Part model, mm, in its own coordinate system. Coordinates: 2 decimals unless noted, no trailing zeros. Write each loop counter-clockwise with the first axis right and the second up, starting at its lowest first coordinate (ties: lowest second). Pieces come first, ordered by that corner, then holes. Notation, with made-up numbers: (27, 30.5) - (56, 30.5) arc R15 cw to (56, 50.5) - close; hole circle Ø10 at (83.5, 61.5). An arc over 180 degrees is marked (long way). Use a Markdown table: item, result.
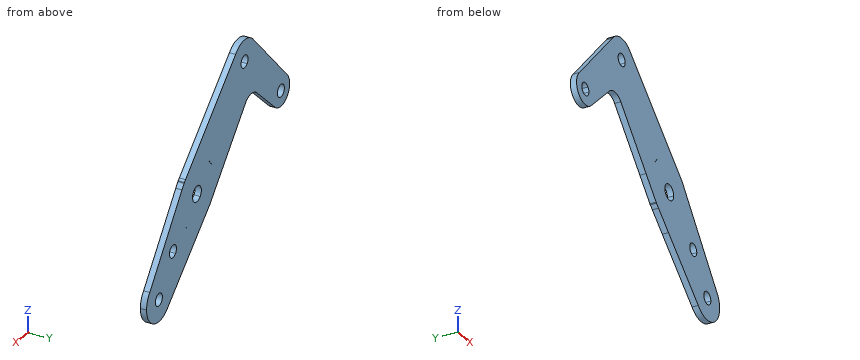
```python
from build123d import *

# Parameters (mm, degrees)
F1_DEPTH = 3.175


with BuildPart() as f1:
    # F0 (on Front) → F1 (new body)
    with BuildSketch(Plane.XZ):
        with BuildLine():
            ThreePointArc((-2.6877932952, 2.9286835289), (1.5995582019, 3.6390704265), (3.9751, 0))
            ThreePointArc((3.9751, 0), (3.6390704265, -1.5995582019), (2.6877932952, -2.9286835289))
            Line((2.6877932952, -2.9286835289), (10.7339987827, -11.6960204828))
            ThreePointArc((10.7339987827, -11.6960204828), (14.5330288597, -6.3880119883), (15.875, 0))
            ThreePointArc((15.875, 0), (15.2734304328, 4.3287351287), (13.5143136611, 8.3294028158))
            Line((13.5143136611, 8.3294028158), (11.6590601378, 10.7741329908))
            Line((11.6590601378, 10.7741329908), (11.4851871667, 10.9592928944))
            Line((11.4851871667, 10.9592928944), (11.3083739877, 11.1416472191))
            Line((11.3083739877, 11.1416472191), (10.3225973322, 12.0606637179))
            ThreePointArc((10.3225973322, 12.0606637179), (-0.2748708071, 15.8726201693), (-10.7339987827, 11.6960204828))
            Line((-10.7339987827, 11.6960204828), (-2.6877932952, 2.9286835289))
        make_face()
        with BuildLine():
            ThreePointArc((-2.9286835289, -2.6877932952), (-3.9714488487, 0.1703351178), (-2.6877932952, 2.9286835289))
            Line((-2.6877932952, 2.9286835289), (-10.7339987827, 11.6960204828))
            Line((-10.7339987827, 11.6960204828), (-13.3268527784, 8.6261590538))
            ThreePointArc((-13.3268527784, 8.6261590538), (-15.8291292061, -1.2059409505), (-11.8662618768, -10.5454944915))
            Line((-11.8662618768, -10.5454944915), (-11.6960204828, -10.7339987827))
            Line((-11.6960204828, -10.7339987827), (-2.9286835289, -2.6877932952))
        make_face()
        with BuildLine():
            Line((10.7339987827, -11.6960204828), (2.6877932952, -2.9286835289))
            ThreePointArc((2.6877932952, -2.9286835289), (-0.1703351178, -3.9714488487), (-2.9286835289, -2.6877932952))
            Line((-2.9286835289, -2.6877932952), (-11.6960204828, -10.7339987827))
            Line((-11.6960204828, -10.7339987827), (-11.5227849075, -10.9197551701))
            Line((-11.5227849075, -10.9197551701), (-9.6887004006, -12.5755600093))
            ThreePointArc((-9.6887004006, -12.5755600093), (-0.5030588817, -15.8670273448), (8.8726348179, -13.1640410357))
            Line((8.8726348179, -13.1640410357), (10.7339987827, -11.6960204828))
        make_face()
        with BuildLine():
            Line((-35.5304524208, 38.714826384), (-10.7339987827, 11.6960204828))
            ThreePointArc((-10.7339987827, 11.6960204828), (-0.2748708071, 15.8726201693), (10.3225973322, 12.0606637179))
            Line((10.3225973322, 12.0606637179), (-34.8667395835, 54.189624641))
            ThreePointArc((-34.8667395835, 54.189624641), (-32.7298053677, 50.7575739011), (-31.9836005106, 46.7840819312))
            ThreePointArc((-31.9836005106, 46.7840819312), (-32.9094460222, 42.3768990566), (-35.5304524208, 38.714826384))
        make_face()
        with BuildLine():
            ThreePointArc((-13.3268527784, 8.6261590538), (-12.1279494046, 10.2434597788), (-10.7339987827, 11.6960204828))
            Line((-10.7339987827, 11.6960204828), (-35.5304524208, 38.714826384))
            ThreePointArc((-35.5304524208, 38.714826384), (-43.4053109787, 35.8417471462), (-51.0052506778, 39.3785392213))
            Line((-51.0052506778, 39.3785392213), (-69.8368422411, 22.0958847311))
            ThreePointArc((-69.8368422411, 22.0958847311), (-68.2881475559, 19.6085836711), (-67.7473524824, 16.7288853397))
            ThreePointArc((-67.7473524824, 16.7288853397), (-68.4183380526, 13.5348793456), (-70.3178530911, 10.8808750983))
            Line((-70.3178530911, 10.8808750983), (-54.0081981098, 25.8490274689))
            ThreePointArc((-54.0081981098, 25.8490274689), (-48.7323738618, 27.7047005709), (-43.6967288942, 25.2715700939))
            Line((-43.6967288942, 25.2715700939), (-20.9173687453, -0.3607843802))
            Line((-20.9173687453, -0.3607843802), (-13.3268527784, 8.6261590538))
        make_face()
        with BuildLine():
            Line((19.3211978133, -21.0528368739), (10.7339987827, -11.6960204828))
            ThreePointArc((10.7339987827, -11.6960204828), (9.830757416, -12.4648238507), (8.8726348179, -13.1640410357))
            Line((8.8726348179, -13.1640410357), (-0.6862483149, -20.7029410933))
            Line((-0.6862483149, -20.7029410933), (26.1615817665, -44.9410646928))
            ThreePointArc((26.1615817665, -44.9410646928), (23.2465029972, -36.9510890975), (26.8349969566, -29.240051207))
            Line((26.8349969566, -29.240051207), (19.3211978133, -21.0528368739))
        make_face()
        with BuildLine():
            ThreePointArc((15.875, 0), (14.5330288597, -6.3880119883), (10.7339987827, -11.6960204828))
            Line((10.7339987827, -11.6960204828), (19.3211978133, -21.0528368739))
            Line((19.3211978133, -21.0528368739), (26.8349969566, -29.240051207))
            ThreePointArc((26.8349969566, -29.240051207), (34.824972552, -26.3249724376), (42.5360104425, -29.9134663971))
            Line((42.5360104425, -29.9134663971), (13.5143136611, 8.3294028158))
            ThreePointArc((13.5143136611, 8.3294028158), (15.2734304328, 4.3287351287), (15.875, 0))
        make_face()
        with BuildLine():
            ThreePointArc((24.8354019053, -18.9060371125), (22.812281241, -21.8647190819), (19.3211978133, -21.0528368739))
            ThreePointArc((19.3211978133, -21.0528368739), (20.5085225697, -15.9473551431), (24.8354019053, -18.9060371125))
        make_face(mode=Mode.SUBTRACT)
        with BuildLine():
            ThreePointArc((-11.8662618768, -10.5454944915), (-15.8291292061, -1.2059409505), (-13.3268527784, 8.6261590538))
            Line((-13.3268527784, 8.6261590538), (-20.9173687453, -0.3607843802))
            Line((-20.9173687453, -0.3607843802), (-11.8662618768, -10.5454944915))
        make_face()
        with BuildLine():
            ThreePointArc((-51.0052506778, 39.3785392213), (-43.4053109787, 35.8417471462), (-35.5304524208, 38.714826384))
            Line((-35.5304524208, 38.714826384), (-40.7891953741, 44.4448778346))
            ThreePointArc((-40.7891953741, 44.4448778346), (-43.0720455442, 43.6119981862), (-45.2751992272, 44.6372821746))
            Line((-45.2751992272, 44.6372821746), (-51.0052506778, 39.3785392213))
        make_face()
        with BuildLine():
            Line((-40.7891953741, 44.4448778346), (-35.5304524208, 38.714826384))
            ThreePointArc((-35.5304524208, 38.714826384), (-32.9094460222, 42.3768990566), (-31.9836005106, 46.7840819312))
            ThreePointArc((-31.9836005106, 46.7840819312), (-32.7298053677, 50.7575739011), (-34.8667395835, 54.189624641))
            ThreePointArc((-34.8667395835, 54.189624641), (-42.4666792826, 57.7264167162), (-50.3415378405, 54.8533374783))
            Line((-50.3415378405, 54.8533374783), (-51.3633206037, 53.7794470598))
            ThreePointArc((-51.3633206037, 53.7794470598), (-53.8850057244, 46.5118413574), (-51.0052506778, 39.3785392213))
            Line((-51.0052506778, 39.3785392213), (-45.2751992272, 44.6372821746))
            ThreePointArc((-45.2751992272, 44.6372821746), (-44.0878744632, 49.7427639018), (-39.7609951306, 46.7840819312))
            ThreePointArc((-39.7609951306, 46.7840819312), (-40.0293893587, 45.5064795335), (-40.7891953741, 44.4448778346))
        make_face()
        with BuildLine():
            Line((-0.6862483149, -20.7029410933), (8.8726348179, -13.1640410357))
            ThreePointArc((8.8726348179, -13.1640410357), (-0.5030588817, -15.8670273448), (-9.6887004006, -12.5755600093))
            Line((-9.6887004006, -12.5755600093), (-0.6862483149, -20.7029410933))
        make_face()
        with BuildLine():
            Line((-69.8368422411, 22.0958847311), (-51.0052506778, 39.3785392213))
            ThreePointArc((-51.0052506778, 39.3785392213), (-53.8850057244, 46.5118413574), (-51.3633206037, 53.7794470598))
            Line((-51.3633206037, 53.7794470598), (-81.0518518738, 22.5768955811))
            ThreePointArc((-81.0518518738, 22.5768955811), (-75.3447264485, 24.6590947021), (-69.8368422411, 22.0958847311))
        make_face()
        with BuildLine():
            ThreePointArc((42.5360104425, -29.9134663971), (34.824972552, -26.3249724376), (26.8349969566, -29.240051207))
            ThreePointArc((26.8349969566, -29.240051207), (23.2465029972, -36.9510890975), (26.1615817665, -44.9410646928))
            ThreePointArc((26.1615817665, -44.9410646928), (38.3803737684, -47.7826524421), (45.4612961045, -37.4272655449))
            ThreePointArc((45.4612961045, -37.4272655449), (44.7041830017, -33.3956878811), (42.5360104425, -29.9134663971))
        make_face()
        with BuildLine():
            ThreePointArc((37.5237961045, -37.4272655449), (33.0711937068, -40.3338713169), (32.201996348, -35.0880614484))
            ThreePointArc((32.201996348, -35.0880614484), (35.6263985022, -34.520659773), (37.5237961045, -37.4272655449))
        make_face(mode=Mode.SUBTRACT)
        with BuildLine():
            ThreePointArc((-67.7473524824, 16.7288853397), (-68.2881475559, 19.6085836711), (-69.8368422411, 22.0958847311))
            Line((-69.8368422411, 22.0958847311), (-73.3456483859, 18.8756850963))
            ThreePointArc((-73.3456483859, 18.8756850963), (-72.7261705118, 17.8807646723), (-72.5098524824, 16.7288853397))
            ThreePointArc((-72.5098524824, 16.7288853397), (-72.7782467105, 15.4512829421), (-73.5380527259, 14.3896812432))
            Line((-73.5380527259, 14.3896812432), (-70.3178530911, 10.8808750983))
            ThreePointArc((-70.3178530911, 10.8808750983), (-68.4183380526, 13.5348793456), (-67.7473524824, 16.7288853397))
        make_face()
        with BuildLine():
            Line((-73.3456483859, 18.8756850963), (-69.8368422411, 22.0958847311))
            ThreePointArc((-69.8368422411, 22.0958847311), (-75.3447264485, 24.6590947021), (-81.0518518738, 22.5768955811))
            ThreePointArc((-81.0518518738, 22.5768955811), (-81.5328627238, 11.3618859484), (-70.3178530911, 10.8808750983))
            Line((-70.3178530911, 10.8808750983), (-73.5380527259, 14.3896812432))
            ThreePointArc((-73.5380527259, 14.3896812432), (-78.8569362274, 16.8649357533), (-73.3456483859, 18.8756850963))
        make_face()
    extrude(amount=F1_DEPTH)


solid = f1.part
```
Item 1: Band-saw the part on A-A, the plane y = -1.75. Count the separate pieces of the cut face and the enclosed holes in it, then the cut area to 3 significant figures.
From the geometry:
| item | result |
|---|---|
| separate pieces | 1 |
| enclosed holes | 7 |
| area | 4,080 mm^2 |
Item 2: Band-saw the part on C-C, the plane x = 6.5. Give the cut face in (y, z) (3 decimals), then the cut area to 3 significant figures.
From the geometry:
| item | result |
|---|---|
| outline | (-3.175, -27.191) - (0, -27.191) - (0, 15.624) - (-3.175, 15.624) - close |
| area | 136 mm^2 |
Item 3: Band-saw the part on B-B, the plane z = 38. Give the cut face in (x, y) (3 decimals).
From the geometry:
| item | result |
|---|---|
| outline | (-66.377, -3.175) - (-17.501, -3.175) - (-17.501, 0) - (-66.377, 0) - close |
Item 4: Drop flat-ended pins along their axis: P1, Ø4, axis at x = 21.66, z = -18.91, coming from the +Y side; P2, Ø1, axis at x = -19, y = -2.5, coming from the -Z side; P3, Ø1.5, axis at y = -2, z = 28.5, coming from the -X side; P4, Ø8.5, axis at x = 34.35, z = -37.43, coming from the +Y side. Give the stop position or say it passes through.
From the geometry:
| item | result |
|---|---|
| P1 | through |
| P2 | z = -3.08 |
| P3 | x = -76.13 |
| P4 | y = 0 |
Item 5: Drill centre lines: probe 1 along Z at (x, y) = (-1, -2.8); probe 2 along X at (y, z) = (-1.55, -35); probe 3 along Z at (x, y) = (-74, -0.4). Where is each one in solid material? Low to high.
From the geometry:
| item | result |
|---|---|
| probe 1 | -20.42 to -3.85, 3.85 to 22.62 |
| probe 2 | 15.15 to 32.3, 36.4 to 45.19 |
| probe 3 | 8.97 to 14.04, 19.42 to 29.99 |
